Verification items for this drawing (mm, ordinates from the low corner). Coordinates: 2 decimals unless noted, no trailing zeros. Order: outer loops, then holes, each group sorted by start corner. A loop starts at its lowest first (then second) coordinate and runs counter-clockwise, first axis right, second up. Notation, with made-up numbers: M 38,-32.5 L 59,-32.5 A18 ccw 59,-27.5 Z; hole C 54.25,-18.75 d1. An arc over 180 degrees is marked long. Write item = value, one per line.
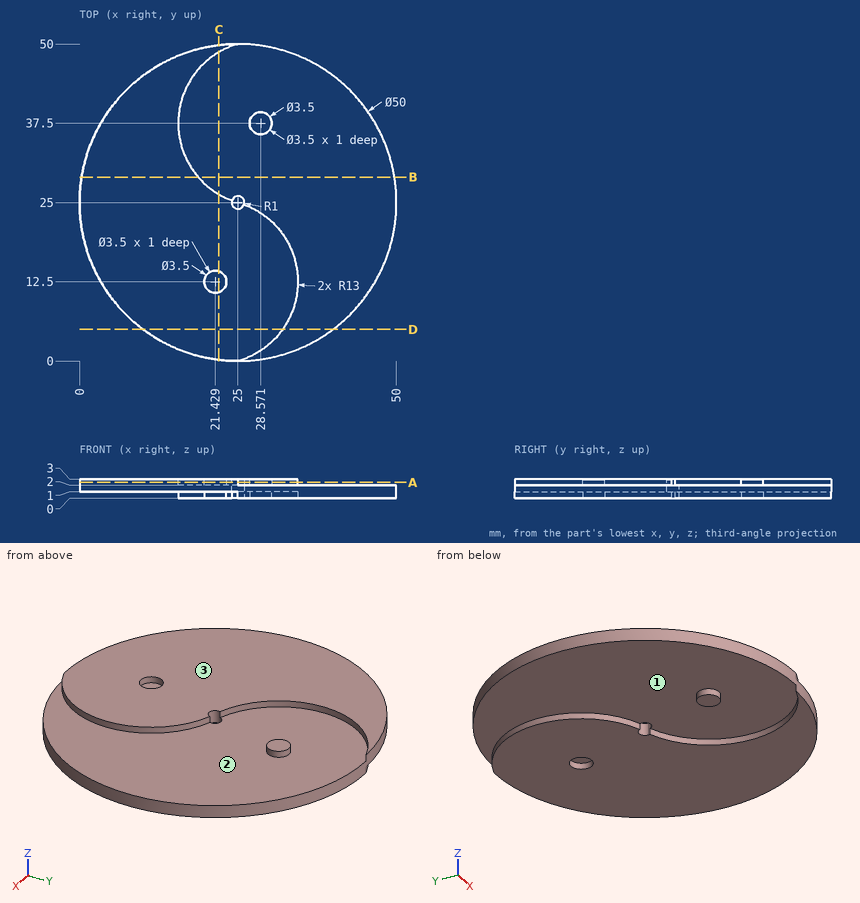
Item 1: Sectioned sample at C-C, the plane x = 22. Enter the section's corners in (y, z).
Report:
outline = M 0.18,1 L 10.85,1 L 10.85,0 L 14.15,0 L 14.15,1 L 26.28,1 L 26.28,0 L 48.72,0 L 48.72,1 L 49.82,1 L 49.82,3 L 48.72,3 L 48.72,2 L 26.28,2 L 26.28,3 L 14.15,3 L 14.15,2 L 10.85,2 L 10.85,3 L 0.18,3 Z
Item 2: Scan lines: L1, parallel to Z at x = 41.5, y = 18; L2, parallel to Z at x = 28.5, y = 10.5; L3, parallel to X at y = 36.5, z = 0.4 (1 decimal). Record each from-to range of solid material in increasing order. Write a range as from..to.
Report:
L1 = 0..2
L2 = 1..3
L3 = 15.6..27.1, 30..47.2
Item 3: Release check for a two-part mould opening along Y. For the marked faces 1, 2 and 3 record: pulls with the +Y half, pulls with the -Y half, needs draft (parallel to the pull), parting line crosses it, or undercut.
Report:
face_1 = undercut
face_2 = undercut
face_3 = needs draft
Item 4: Gauge pin test, flat ends, axial feed: pin 1 (17 mm diameter, centred on x = 24.5, y = 36.5, fed in from +Z); pin 2 (1 mm diameter, centred on x = 9.5, y = 44.5, fed in from -Z); pin 3 (1 mm diameter, centred on x = 35.5, z = 0.5, fed in from +Y); pin 4 (3 mm diameter, centred on x = 33.5, y = 42, fed in from +Z). Record the tip position at first contact, or that the pin passes through.
Report:
pin_1 = 3
pin_2 = 1
pin_3 = 47.91
pin_4 = 2
Item 5: Sectioned sample at D-D, the plane y = 5. Enter the section's corners in (x, z).
Report:
outline = M 10,1 L 32.05,1 L 32.05,0 L 40,0 L 40,2 L 32.05,2 L 32.05,3 L 10,3 Z
Item 6: Sectioned sample at A-A, the plane z = 2.45. Enter the section's corners in (x, y), then the cut area to 3 significant figures.
Report:
outline = M 24.05,25.31 A13 cw 25,50 A25 ccw 25,0 A13 ccw 25.95,24.69 A1 cw Z; C 28.57,37.5 d3.5; hole C 21.43,12.5 d3.5
area = 980 mm^2
Item 7: Sectioned sample at B-B, the plane y = 29. Enter the section's corners in (x, z) (1 decimal).
Report:
outline = M 0.3,1 L 18.7,1 L 18.7,0 L 49.7,0 L 49.7,2 L 18.7,2 L 18.7,3 L 0.3,3 Z
